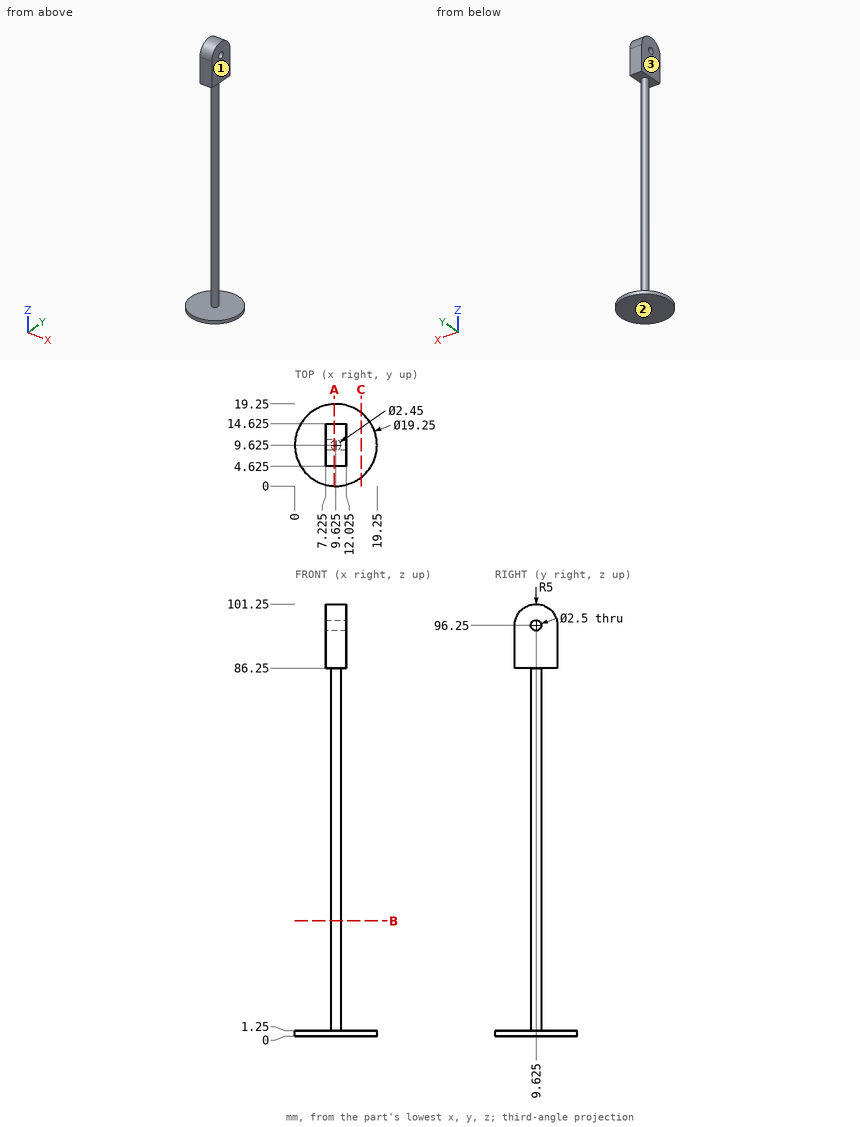
Here's the drawing with two shaded views (mm, measured from the low corner). I have some questions. A direction names the side the tool comes from. Give positions to 0.01 mm unless a question says otherwise; leave off trailing zeros. Write each loop counter-clockwise with the first axis right and the second up, starting at its lowest first coordinate (ties: lowest second). Pieces come first, ordered by that corner, then holes. Notation, with made-up numbers: (43.25, 75) -> (95.25, 75) arc R30 cw to (95.25, 113) -> close; hole circle Ø8 at (40.5, 72). An arc over 180 degrees is marked (long way). Use one line per item in the form item = value.
1) On a 3-axis mill with a long thin cutter (end or side, diameter ignored), from which of +Z, -Z, +X, -X, +Y, -Y can I reach the whole of each face in a straight line? I mean the marked faces 1, 2 and 3. Say none if no direction works.
Verdict:
face_1 = +Z, +X, +Y, -Y
face_2 = -Z, +X, -X, +Y, -Y
face_3 = +Z, -X, +Y, -Y
2) I'm going to push flat-ended pins straight in: pin 1 (6 mm diameter, centred on x = 9, z = 15.5, fed in from -Y); pin 2 (5 mm diameter, centred on x = 5, z = 18.5, fed in from -Y); pin 3 (3 mm diameter, centred on y = 11, z = 93, fed in from +X) (3 decimals); pin 4 (5 mm diameter, centred on y = 10, z = 91, fed in from -X) (3 decimals). Where does each tip first touch, or does it pass through?
Verdict:
pin_1 = 8.4
pin_2 = through
pin_3 = 12.025
pin_4 = 7.225
3) Suppose I cut it at C-C (x = 15.5). Please give me the cut outline in (y, z).
Verdict:
outline = (2, 0) -> (17.25, 0) -> (17.25, 1.25) -> (2, 1.25) -> close
4) If I drill on L1, parallel to Y at x = 10.85, z = 96.25 (3 decimals); L2, parallel to Z at x = 8.5, y = 1.75; L3, parallel to Z at x = 9.25, y = 12.5, over which ranges is the centre line in solid material (lowest first)? Write a range as [from, to].
Verdict:
L1 = [4.625, 8.375], [10.875, 14.625]
L2 = [0, 1.25]
L3 = [0, 1.25], [86.25, 100.34]
5) Suppose I cut it at A-A (x = 9.25). Please give me the cut outline in (y, z) (3 decimals), and give its area (3 significant figures).
Verdict:
outline = (0.007, 0) -> (19.243, 0) -> (19.243, 1.25) -> (10.791, 1.25) -> (10.791, 86.25) -> (14.625, 86.25) -> (14.625, 96.25) arc R5 ccw to (4.625, 96.25) -> (4.625, 86.25) -> (8.459, 86.25) -> (8.459, 1.25) -> (0.007, 1.25) -> close; hole circle Ø2.5 at (9.625, 96.25)
area = 357 mm2
6) Suppose I cut it at B-B (z = 27). Please give me the cut outline in (x, y) (3 decimals).
Verdict:
outline = circle Ø2.45 at (9.625, 9.625)
